Here's how the part is built. I have some questions about the finished solid (model axes, mm). Face numbers are marked on the shaded views. A direction names the side the tool comes from. Coordinates: 2 decimals unless noted, no trailing zeros. Order: outer loops, then holes, each group sorted by start corner. A loop starts at its lowest first (then second) coordinate and runs counter-clockwise, first axis right, second up. Notation, with made-up numbers: (16, 73) - (74, 73) arc R26 ccw to (74, 93) - close; hole circle Ø5 at (27, 34.5). An arc over 180 degrees is marked (long way). Use one line per item in the form item = value. Start each with the question number.
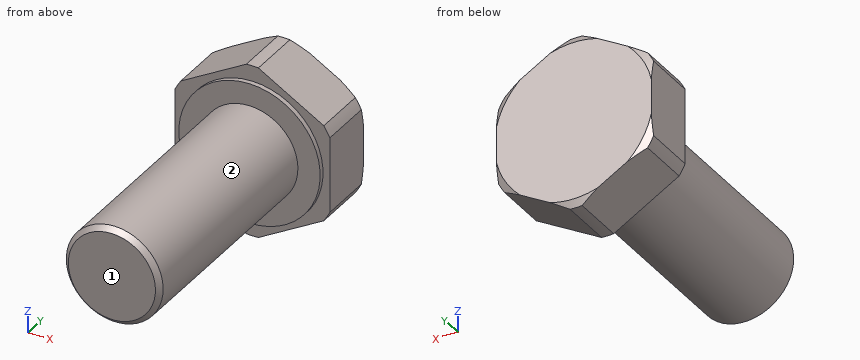
from build123d import *

# Parameters (mm, degrees)
SZKIC2_OUTSIDE_W           = 27.694
SZKIC2_OUTSIDE_H           = 27.694
WYTNIJ_WYCI_GNI_CIE1_DEPTH = 30.4


with BuildPart() as part:
    # Szkic1 → Obrót1 (revolve)
    with BuildSketch(Plane.XY, mode=Mode.PRIVATE) as obr_t1_sk:
        Polygon((0, 6.4), (8.2, 6.4), (8.9, 5.995854812), (8.9, 0.5), (7.3, 0.5), (7.3, 0), (5, 0), (5, -23.5), (4.5, -24), (0, -24), align=None)
    revolve(obr_t1_sk.sketch.rotate(Axis((0, 37.287865055, 0), (0, -1, 0)), 90), axis=Axis((0, 37.287865055, 0), (0, -1, 0)))

    # Szkic2 outside → Wytnij-wyciągnięcie1 (cut)
    with BuildSketch(Plane(origin=(0, 6.4, 0), x_dir=(1, 0, 0), z_dir=(0, 1, 0))):
        Rectangle(SZKIC2_OUTSIDE_W, SZKIC2_OUTSIDE_H)
        Polygon((0, 9.237604307), (-8, 4.618802154), (-8, -4.618802154), (0, -9.237604307), (8, -4.618802154), (8, 4.618802154), align=None, mode=Mode.SUBTRACT)
    extrude(amount=-WYTNIJ_WYCI_GNI_CIE1_DEPTH, mode=Mode.SUBTRACT)


solid = part.part
1) I need wall thicknesses on probe 1 along Y at (x, z) = (-2.5, -5.25); probe 2 along X at (y, z) = (-21.5, 0); probe 3 along Y at (x, z) = (4.25, 6.5). Which ranges of each line are inside material? Lowest first, please. Write a range as [from, to].
2) Suppose I cut it at A-A, the plane x = 0. List the corners of the cut face in (y, z) for me, then the cut area to 3 significant figures.
3) Which directions (+Z, -Z, +X, -X, +Y, -Y) give clear straight access to the entire face, cutting with the end or side of a thin tool? Please do the marked faces 1 and 2.
4) Suppose I cut it at C-C, the plane y = -5. List the corners of the cut face in (x, z) for me, then the cut area to 3 significant figures.
5) For pin 1 (5 mm diameter, centred on x = -2, y = -17, fed in from -Z); pin 2 (10 mm diameter, centred on y = -21, z = -5, fed in from +X); pin 3 (2 mm diameter, centred on x = -1.5, z = -6.5, fed in from -Y), each with a flat end and sliding along its axis, tell me the tip position at first contact or that it passes through.
6) Suppose I cut it at B-B, the plane z = 0. List the corners of the cut face in (x, y) for me, then the cut area to 3 significant figures.
From the geometry:
q1.probe_1 = [0, 6.4]
q1.probe_2 = [-5, 5]
q1.probe_3 = [0.5, 6.4]
q2.outline = (-24, -4.5) - (-23.5, -5) - (0, -5) - (0, -7.3) - (0.5, -7.3) - (0.5, -8.9) - (6, -8.9) - (6.4, -8.2) - (6.4, 8.2) - (6, 8.9) - (0.5, 8.9) - (0.5, 7.3) - (0, 7.3) - (0, 5) - (-23.5, 5) - (-24, 4.5) - close
q2.area = 352 mm2
q3.face_1 = +Z, -Z, +X, -X, -Y
q3.face_2 = -Y
q4.outline = circle Ø10 at (0, 0)
q4.area = 78.5 mm2
q5.pin_1 = -5
q5.pin_2 = 5
q5.pin_3 = 0
q6.outline = (-8, 0.5) - (-7.3, 0.5) - (-7.3, 0) - (-5, 0) - (-5, -23.5) - (-4.5, -24) - (4.5, -24) - (5, -23.5) - (5, 0) - (7.3, 0) - (7.3, 0.5) - (8, 0.5) - (8, 6.4) - (-8, 6.4) - close
q6.area = 341 mm2
